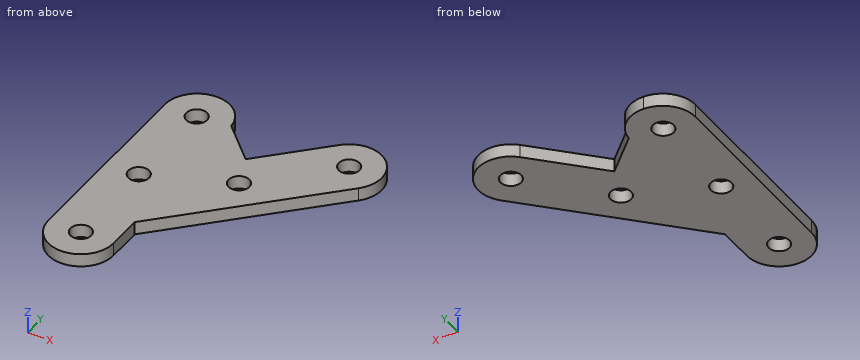
from build123d import *

# Parameters (mm, degrees)
EXTRUDE_1_DEPTH     = 1
FILLET_1_R          = 5
SKETCH_2_R          = 1.6
CUT_EXTRUDE_1_DEPTH = 36.923820844


with BuildPart() as part:
    # ｽｹｯﾁ1 → ﾎﾞｽ - 押し出し1 (new, symmetric)
    with BuildSketch(Plane.XY):
        Polygon((-3.827856705, 20.364933264), (-3.827856705, -19.777202359), (6.172143295, -19.777202359), (6.172143295, -9.277202359), (31.274434027, 15.825088373), (24.203366215, 22.896156185), (11.601075483, 10.293865452), (6.172143295, 15.722797641), (6.172143295, 20.364933264), align=None)
    extrude(amount=EXTRUDE_1_DEPTH, both=True)

    # ﾌｨﾚｯﾄ1
    # the kernel refuses this fillet: 5 mm, written as the material it takes off along each edge
    with BuildSketch(Plane(origin=(24.203366215, 22.896156185, -13.5), x_dir=(-0.7071067811865422, -0.7071067811865529, 0), z_dir=(0, 0, 1)), Plane(origin=(-3.827856705, -19.777202359, -13.5), x_dir=(1, 0, 0), z_dir=(0, 0, 1)), Plane(origin=(6.172143295, -19.777202359, -13.5), x_dir=(0, 1, 0), z_dir=(0, 0, 1)), Plane(origin=(31.274434027, 15.825088373, -13.5), x_dir=(-0.7071067811865479, 0.7071067811865471, 0), z_dir=(0, 0, 1))) as fillet_1_piece_1:
        with BuildLine():
            CenterArc((FILLET_1_R, FILLET_1_R), FILLET_1_R, 180, 90)
            Line((0, FILLET_1_R), (-FILLET_1_R * 0.02, FILLET_1_R))
            Line((-FILLET_1_R * 0.02, FILLET_1_R), (-FILLET_1_R * 0.02, -FILLET_1_R * 0.02))
            Line((-FILLET_1_R * 0.02, -FILLET_1_R * 0.02), (FILLET_1_R, -FILLET_1_R * 0.02))
            Line((FILLET_1_R, -FILLET_1_R * 0.02), (FILLET_1_R, 0))
        make_face()
    extrude(amount=27, mode=Mode.SUBTRACT)
    with BuildSketch(Plane(origin=(-3.827856705, 20.364933264, -13.5), x_dir=(1, 0, 0), z_dir=(0, 0, 1))) as fillet_1_piece_2:
        with BuildLine():
            CenterArc((FILLET_1_R, -FILLET_1_R), FILLET_1_R, 90, 90)
            Line((0, -FILLET_1_R), (-FILLET_1_R * 0.02, -FILLET_1_R))
            Line((-FILLET_1_R * 0.02, -FILLET_1_R), (-FILLET_1_R * 0.02, FILLET_1_R * 0.02))
            Line((-FILLET_1_R * 0.02, FILLET_1_R * 0.02), (FILLET_1_R, FILLET_1_R * 0.02))
            Line((FILLET_1_R, FILLET_1_R * 0.02), (FILLET_1_R, 0))
        make_face()
    extrude(amount=27, mode=Mode.SUBTRACT)
    with BuildSketch(Plane(origin=(6.172143295, 20.364933264, 13.467942164), x_dir=(-1, 0, 0), z_dir=(0, 0, -1))) as fillet_1_piece_3:
        with BuildLine():
            CenterArc((4.987176866, -5), FILLET_1_R, 90, 85.895667026)
            Line((0, -4.642135624), (-0.099743537, -4.634978336))
            ThreePointArc((-0.099743537, -4.634978336), (-0.1, -2.321067812), (-0.1, 0))
            Line((-0.1, 0), (0, 0.1))
            Line((0, 0.1), (4.987176866, 0.1))
            Line((4.987176866, 0.1), (4.987176866, 0))
        make_face()
    extrude(amount=26.935884328, mode=Mode.SUBTRACT)

    # ｽｹｯﾁ2 → ｶｯﾄ - 押し出し1 (cut, through all)
    with BuildSketch(Plane.XY.offset(1)):
        with Locations((1.171422694, -14.777202359)):
            Circle(SKETCH_2_R)
        with Locations((13.596764497, 5.218486655)):
            Circle(SKETCH_2_R)
        with Locations((24.203366215, 15.825088373)):
            Circle(SKETCH_2_R)
        with Locations((1.171422694, 0.222797641)):
            Circle(SKETCH_2_R)
        with Locations((1.171422694, 15.222797641)):
            Circle(SKETCH_2_R)
    extrude(amount=-CUT_EXTRUDE_1_DEPTH, mode=Mode.SUBTRACT)


solid = part.part
Geometry: final body of the model. Coordinates: model frame, mm. Round coordinates to 2 decimals unless told otherwise and drop trailing zeros. Order: outer loops, then holes, each group sorted by start corner. A loop starts at its lowest first (then second) coordinate and runs counter-clockwise, first axis right, second up. Notation, with made-up numbers: (17, 49) - (56, 49) arc R24 cw to (56, 85) - close; hole circle Ø1 at (-14.75, -40). An arc over 180 degrees is marked (long way). Write each question's results on one line, items separated by ' | '.
Item 1: Section B-B, the plane x = 13. Return the cut outline in (y, z), and give its area (3 significant figures).
Completed:
outline: (-2.45, -1) - (3.73, -1) - (3.73, 1) - (-2.45, 1) - close; (6.7, -1) - (11.69, -1) - (11.69, 1) - (6.7, 1) - close | area: 22.3 mm^2
Item 2: Section C-C, the plane z = 0.1. State how many separate pieces and enclosed holes the cut face has, and give its area (3 significant figures).
Completed:
separate pieces: 1 | enclosed holes: 5 | area: 664 mm^2
Item 3: Section A-A, the plane y = 1. Return the cut outline in (x, z).
Completed:
outline: (-3.83, -1) - (-0.23, -1) - (-0.23, 1) - (-3.83, 1) - close; (2.57, -1) - (16.45, -1) - (16.45, 1) - (2.57, 1) - close
Item 4: First-contact query: pin 1 Ø1 at (y, z) = (-11.5, 0) entering from +X; pin 2 Ø1 at (y, z) = (14, -0.5) entering from +X. Flat tips, straight axial feed; report the tip coordinate or a pass-through.
Completed:
pin 1: x = 6.17 | pin 2: x = 29.02
Item 5: Section D-D, the plane y = -12. Return the cut outline in (x, z).
Completed:
outline: (-3.83, -1) - (6.17, -1) - (6.17, 1) - (-3.83, 1) - close
Item 6: Material intervals for line 1 along Y through (x, z) = (1, -0.1); line 2 along Y through (x, z) = (0, -0.55); line 3 along X through (y, z) = (-10, -0.65), sorted ascending. Write a range as [from, to].
Completed:
line 1: [-19.77, -16.37], [-13.19, -1.37], [1.81, 13.63], [16.81, 20.36] | line 2: [-19.64, -15.87], [-13.69, -0.87], [1.31, 14.13], [16.31, 20.23] | line 3: [-3.83, 6.17]
